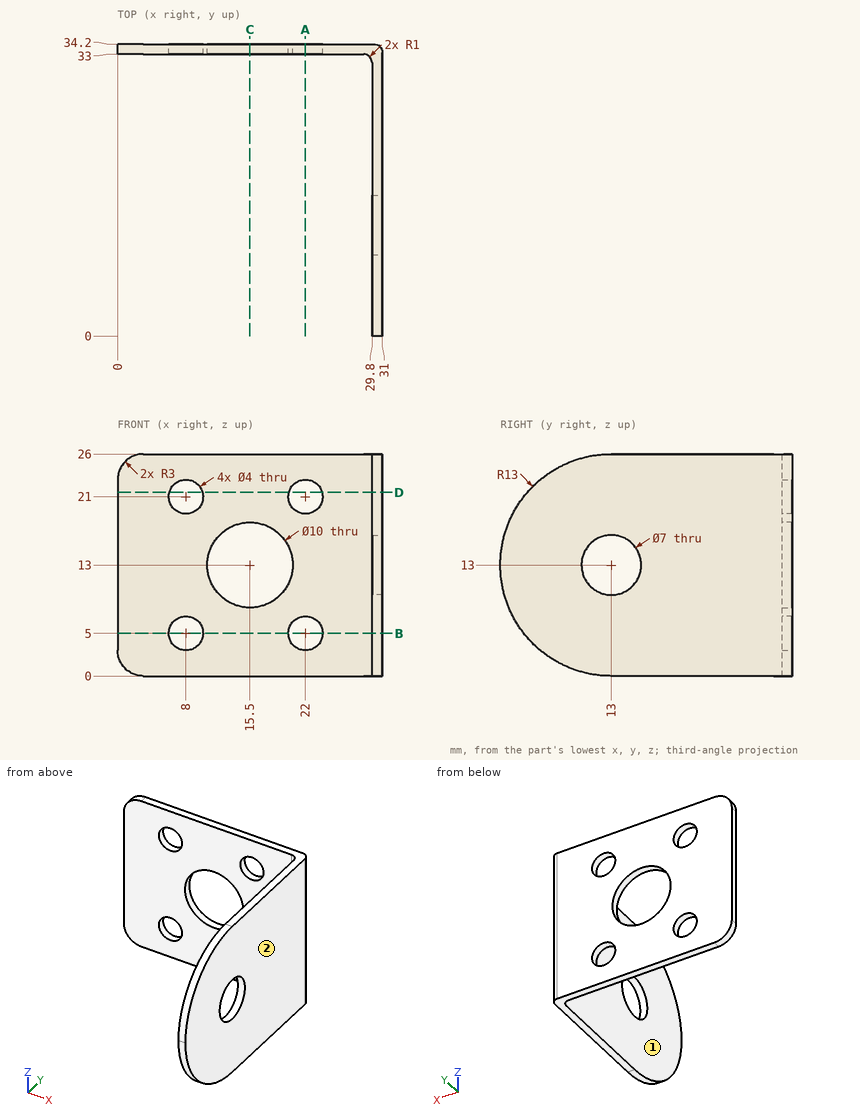
Design review of the part shown in the three views and the two pictorial views. Dimensions are in mm from the part's minimum x, y and z. A direction names the side the tool comes from. Give positions to 0.01 mm unless a question says otherwise; leave off trailing zeros. Loops run counter-clockwise (first coordinate to the right, second up) from the corner with the lowest first, then second, coordinate; pieces in that order, holes last. Notation, with made-up numbers: (17, 58) - (51, 58) arc R25 ccw to (51, 77) - close; hole circle Ø8 at (35, 2.5). An arc over 180 degrees is marked (long way). Answer as a JSON object with one key per item and string values.
Q1. To check wall thickness, follow line 1 along X through (y, z) = (5.5, 22.5); line 2 along Y through (x, z) = (21, 2.5); line 3 along X through (y, z) = (33.55, 5). State the ranges of each line that lie inside material, in increasing order.
Worked out:
{"line 1": "x = 29.8 to 31", "line 2": "y = 33 to 34.2", "line 3": "x = 0 to 6, 10 to 20, 24 to 30.94"}
Q2. Add section B-B on z = 5. State the section outline as (x, y) points, plus the area to 3 significant figures.
Worked out:
{"outline": "(0, 33) - (6, 33) - (6, 34.2) - (0, 34.2) - close; (10, 33) - (20, 33) - (20, 34.2) - (10, 34.2) - close; (24, 33) - (28.8, 33) arc R1 cw to (29.8, 32) - (29.8, 2.75) - (31, 2.75) - (31, 33.2) arc R1 ccw to (30, 34.2) - (24, 34.2) - close", "area": "63.9 mm^2"}
Q3. For the marked faces 1 and 2, list the 3-axis set-ups (+Z, -Z, +X, -X, +Y, -Y) from which the entire face can be reached by the end or side of a thin tool; tool diameter is ignored.
Worked out:
{"face 1": "+Z, -Z, -X, -Y", "face 2": "+Z, -Z, +X, +Y, -Y"}
Q4. Insertion check: pin 1 (8 mm diameter, centred on y = 11, z = 6.5, fed in from -X); pin 2 (6.5 mm diameter, centred on x = 22, z = 21, fed in from -Y). Each pin has a flat end and moves straight along its axis. Give the tip position at first contact, or say it passes through.
Worked out:
{"pin 1": "stops at x = 29.8", "pin 2": "stops at y = 33"}
Q5. Add section A-A on x = 22. State the section outline as (y, z) points, plus the area to 3 significant figures.
Worked out:
{"outline": "(33, 0) - (34.2, 0) - (34.2, 3) - (33, 3) - close; (33, 7) - (34.2, 7) - (34.2, 19) - (33, 19) - close; (33, 23) - (34.2, 23) - (34.2, 26) - (33, 26) - close", "area": "21.6 mm^2"}
Q6. Add section C-C on x = 15.5. State the section outline as (y, z) points, plus the area to 3 significant figures.
Worked out:
{"outline": "(33, 0) - (34.2, 0) - (34.2, 8) - (33, 8) - close; (33, 18) - (34.2, 18) - (34.2, 26) - (33, 26) - close", "area": "19.2 mm^2"}
Q7. Add section D-D on z = 21.5. State the section outline as (x, y) points, plus the area to 3 significant figures.
Worked out:
{"outline": "(0, 33) - (6.06, 33) - (6.06, 34.2) - (0, 34.2) - close; (9.94, 33) - (20.06, 33) - (20.06, 34.2) - (9.94, 34.2) - close; (23.94, 33) - (28.8, 33) arc R1 cw to (29.8, 32) - (29.8, 3.16) - (31, 3.16) - (31, 33.2) arc R1 ccw to (30, 34.2) - (23.94, 34.2) - close", "area": "63.7 mm^2"}
